```python
from build123d import *

# Parameters (mm, degrees)
SKETCH_2_W                = 45
SKETCH_2_H                = 65
SKETCH_2_R                = 2.25
SKETCH_2_R_2              = 1.75
EXTRUDE_1_DEPTH           = 7
HOLE_WIZARD_1_D           = 4.5
HOLE_WIZARD_1_CBORE_D     = 7.3
HOLE_WIZARD_1_CBORE_DEPTH = 4.2
CUT_EXTRUDE_1_DEPTH       = 2.5


with BuildPart() as part:
    # 草圖2 → 填料-伸長1 (new body)
    with BuildSketch(Plane.XY):
        Rectangle(SKETCH_2_W, SKETCH_2_H)
        with Locations((-18, 18)):
            Circle(SKETCH_2_R, mode=Mode.SUBTRACT)
        with Locations((-17.5, 28.5)):
            Circle(SKETCH_2_R_2, mode=Mode.SUBTRACT)
        with Locations((18, 18)):
            Circle(SKETCH_2_R, mode=Mode.SUBTRACT)
        with Locations((18, -18)):
            Circle(SKETCH_2_R, mode=Mode.SUBTRACT)
        with Locations((-18, -18)):
            Circle(SKETCH_2_R, mode=Mode.SUBTRACT)
        with Locations((17.5, 28.5)):
            Circle(SKETCH_2_R_2, mode=Mode.SUBTRACT)
        with Locations((17.5, -28.5)):
            Circle(SKETCH_2_R_2, mode=Mode.SUBTRACT)
        with Locations((-17.5, -28.5)):
            Circle(SKETCH_2_R_2, mode=Mode.SUBTRACT)
    extrude(amount=EXTRUDE_1_DEPTH)

    # 鑽孔1 (through all)
    with Locations(Plane(origin=(-18, 18, 7), x_dir=(1, 0, 0), z_dir=(0, 0, 1))):
        with Locations((0, 0), (36, 0), (36, -36), (0, -36)):
            CounterBoreHole(HOLE_WIZARD_1_D / 2, HOLE_WIZARD_1_CBORE_D / 2, HOLE_WIZARD_1_CBORE_DEPTH)

    # 草圖4 → 除料-伸長1 (cut)
    with BuildSketch(Plane(origin=(0, 0, 0), x_dir=(-1, 0, 0), z_dir=(0, 0, -1))):
        Polygon((-14.209103466, 28.5), (-15.854551733, 31.35), (-19.145448267, 31.35), (-20.790896534, 28.5), (-19.145448267, 25.65), (-15.854551733, 25.65), align=None)
        Polygon((15.854551733, 25.65), (14.209103466, 28.5), (15.854551733, 31.35), (19.145448267, 31.35), (20.790896534, 28.5), (19.145448267, 25.65), align=None)
        Polygon((14.209103466, -28.5), (15.854551733, -31.35), (19.145448267, -31.35), (20.790896534, -28.5), (19.145448267, -25.65), (15.854551733, -25.65), align=None)
        Polygon((-15.854551733, -25.65), (-14.209103466, -28.5), (-15.854551733, -31.35), (-19.145448267, -31.35), (-20.790896534, -28.5), (-19.145448267, -25.65), align=None)
    extrude(amount=-CUT_EXTRUDE_1_DEPTH, mode=Mode.SUBTRACT)


solid = part.part
```
Part model, mm, in its own coordinate system. A direction names the side the tool comes from. Round coordinates to 2 decimals unless told otherwise and drop trailing zeros. Write each loop counter-clockwise with the first axis right and the second up, starting at its lowest first coordinate (ties: lowest second). Pieces come first, ordered by that corner, then holes. Notation, with made-up numbers: (41.25, 77.5) -> (51.25, 77.5) arc R22 ccw to (51.25, 95.5) -> close; hole circle Ø1 at (65, 73.5). An arc over 180 degrees is marked (long way). Return JSON: item names as keys, results as strings. Group by question number.
Q1. Probe L1, parallel to Y at x = -18, z = 1.6; L2, parallel to X at y = 28.5, z = 4.7; L3, parallel to Y at x = -17.5, z = 3.85. List the from-to ranges inside material, lowest first. Write a range as [from, to].
Q2. Mould opens along X. For faces 1 (the flat face through (22.5, 0, 3)), 2 (the flat face through (0, -32.5, 3)), 3 (the cylindrical face through (-21.646, -17.84, 4.929)) say: pulls with the +X half, pulls with the -X half, needs draft (parallel to the pull), parting line crosses it, or undercut.
Q3. Saw through at A-A on z = 1.25. State how many separate pieces and enclosed holes the cut face has, plus the area to 3 significant figures.
Q4. Saw through at B-B on y = -18. Write the cut outline in (x, z).
Q5. Pin check, flat tip, straight feed: pin 1 (3.5 mm diameter, centred on x = -16.5, y = -17, fed in from +Z). Stop position of the tip, or through.
Q6. Which spindle directions (+Z, -Z, +X, -X, +Y, -Y) get a long thin tool onto all of the face, cutting with end or side? Do faces 4 (the cylindrical face through (19.038, 16.004, 1.38)), 5 (the cylindrical face through (14.354, 18.16, 4.929)), 6 (the flat face through (-15.04, 27.06, 1.23)). Say none if no direction does.
Answer:
{
 "1": {"L1": "[-32.5, -31.35], [-25.65, -20.25], [-15.75, 15.75], [20.25, 25.65], [31.35, 32.5]", "L2": "[-22.5, -19.25], [-15.75, 15.75], [19.25, 22.5]", "L3": "[-32.5, -30.25], [-26.75, -21.62], [-14.38, 14.38], [21.62, 26.75], [30.25, 32.5]"},
 "2": {"face 1": "pulls with the +X half", "face 2": "needs draft", "face 3": "undercut"},
 "3": {"separate pieces": "1", "enclosed holes": "8", "area": "2,750 mm2"},
 "4": {"outline": "(-22.5, 0) -> (-20.25, 0) -> (-20.25, 2.8) -> (-21.65, 2.8) -> (-21.65, 7) -> (-22.5, 7) -> close; (-15.75, 0) -> (15.75, 0) -> (15.75, 2.8) -> (14.35, 2.8) -> (14.35, 7) -> (-14.35, 7) -> (-14.35, 2.8) -> (-15.75, 2.8) -> close; (20.25, 0) -> (22.5, 0) -> (22.5, 7) -> (21.65, 7) -> (21.65, 2.8) -> (20.25, 2.8) -> close"},
 "5": {"pin 1": "z = 2.8"},
 "6": {"face 4": "+Z, -Z", "face 5": "+Z", "face 6": "-Z"}
}
